Autodesk Inventor part; units mm, degrees
ref_plane "YZ Plane" through (0, 0, 0) normal (1, 0, 0) x (0, 1, 0)
ref_plane "XZ Plane" through (0, 0, 0) normal (0, 1, 0) x (-1, 0, 0)
ref_plane "XY Plane" through (0, 0, 0) normal (0, 0, 1) x (1, 0, 0)
sketch "Sketch1" plane through (0, 0, 0) normal (0, 0, 1) x (1, 0, 0)
  circle A0 centre (0, 0) radius 10
  line L0 (0, 0) -> (-140, 0)
  line L1 (0, 0) -> (140, 0) construction
  circle A1 centre (-140, 0) radius 10
  dimension "d0" = 20
  dimension "d1" = 140
  dimension "d2" = 180
  dimension "d3" = 20
sketch "Sketch2" plane through (0, 0, 0) normal (0, 1, 0) x (-1, 0, 0)
  line L0 (0, 0) -> (0, 20)
  line L1 (20, 40) -> (120, 40)
  line L2 (140, 20) -> (140, 0)
  arc A0 (140, 20) -> (120, 40) centre (120, 20) ccw
  arc A1 (20, 40) -> (0, 20) centre (20, 20) ccw
  point P0 (0, 40)
  point P1 (140, 40)
  dimension "d4" = 40
  dimension "d5" = 140
  dimension "d6" = 20
sweep "Sweep1" add profiles "Sketch1" path "Sketch2" path curves L2 A0 L1 A1 contours A1
extrude "Extrusion1" add sketch "Sketch1" along normal up to surface (20 mm away) contours A0
properties part number "handle_140_20"
Geometry check sheet. Reference: the model listing, model coordinates, mm. A direction names the side the tool comes from. Round coordinates to 2 decimals unless told otherwise and drop trailing zeros. Loops run counter-clockwise (first coordinate to the right, second up) from the corner with the lowest first, then second, coordinate; pieces in that order, holes last. Notation, with made-up numbers: (61.25, -19.75) - (96.25, -19.75) arc R30 ccw to (96.25, 16.25) - close; hole circle Ø7 at (87, 0.5). An arc over 180 degrees is marked (long way). Use a Markdown table: item, result.
Q1. Material ranges on line 1 (Z direction, x = -79, y = -0.5); line 2 (X direction, y = -3.5, z = 13); line 3 (X direction, y = 4.5, z = 16), recorded low to high.
Solutions:
| item | result |
|---|---|
| line 1 | z = 30.01 to 49.99 |
| line 2 | x = -149.37 to -130.63, -9.37 to 9.37 |
| line 3 | x = -148.93 to -131.07, -8.93 to 8.93 |
Q2. Cross-section at B-B on y = 5.5. Record the cut outline in (x, z), plus the area to 3 significant figures.
Solutions:
| item | result |
|---|---|
| outline | (-148.35, 0) - (-131.65, 0) - (-131.65, 20) arc R11.65 cw to (-120, 31.65) - (-20, 31.65) arc R11.65 cw to (-8.35, 20) - (-8.35, 0) - (8.35, 0) - (8.35, 20) arc R28.35 ccw to (-20, 48.35) - (-120, 48.35) arc R28.35 ccw to (-148.35, 20) - close |
| area | 3,390 mm2 |
Q3. Draft check along X on faces 3 (the cylindrical face through (-130.763, 3.83, 9.86)), 4 (the flat face through (-140, 0, 0)), 5 (the cylindrical face through (-2.17, 9.76, 9.86)). Enter one of: released by +X, released by -X, zero draft, split by the parting line, or undercut.
Solutions:
| item | result |
|---|---|
| face 3 | undercut |
| face 4 | zero draft |
| face 5 | undercut |
Q4. Access from +Z, -Z, +X, -X, +Y, -Y to the whole of each face (thin tool, end or side, straight path). Record for faces 1 (the cylindrical face through (-71, 0, 50)), 2 (the flat face through (0, 0, 0)).
Solutions:
| item | result |
|---|---|
| face 1 | none |
| face 2 | -Z, +X, -X, +Y, -Y |
Q5. Cross-section at C-C on x = -105. Record the cut outline in (y, z).
Solutions:
| item | result |
|---|---|
| outline | circle Ø20 at (0, 40) |
Q6. Cross-section at A-A on z = 5. Record the cut outline in (x, y), plus the area to 3 significant figures.
Solutions:
| item | result |
|---|---|
| outline | circle Ø20 at (-140, 0); circle Ø20 at (0, 0) |
| area | 628 mm2 |
Q7. Go/stop test with flat-tipped pins: P1, Ø12, axis at x = -26, y = -3.5, coming from the -Z side; P2, Ø8, axis at x = -64.5, z = 30, coming from the +Y side; P3, Ø6, axis at y = -3.5, z = 44.5, coming from the +X side; P4, Ø4, axis at x = -74.5, y = 1.5, coming from the +Z side. Record where each tip stops, or that it passes through.
Solutions:
| item | result |
|---|---|
| P1 | stops at z = 30 |
| P2 | stops at y = 8 |
| P3 | stops at x = 0.28 |
| P4 | stops at z = 50 |
Q8. Cross-section at D-D on y = -8.25. Record the cut outline in (x, z), plus the area to 3 significant figures.
Solutions:
| item | result |
|---|---|
| outline | (-145.65, 0) - (-134.35, 0) - (-134.35, 20) arc R14.35 cw to (-120, 34.35) - (-20, 34.35) arc R14.35 cw to (-5.65, 20) - (-5.65, 0) - (5.65, 0) - (5.65, 20) arc R25.65 ccw to (-20, 45.65) - (-120, 45.65) arc R25.65 ccw to (-145.65, 20) - close |
| area | 2,290 mm2 |
